The drawing under review shows one solid part. Ordinate dimensions are in mm from its lowest x, y, z. A direction names the side the tool comes from. Round coordinates to 2 decimals unless told otherwise and drop trailing zeros. Order: outer loops, then holes, each group sorted by start corner. A loop starts at its lowest first (then second) coordinate and runs counter-clockwise, first axis right, second up.
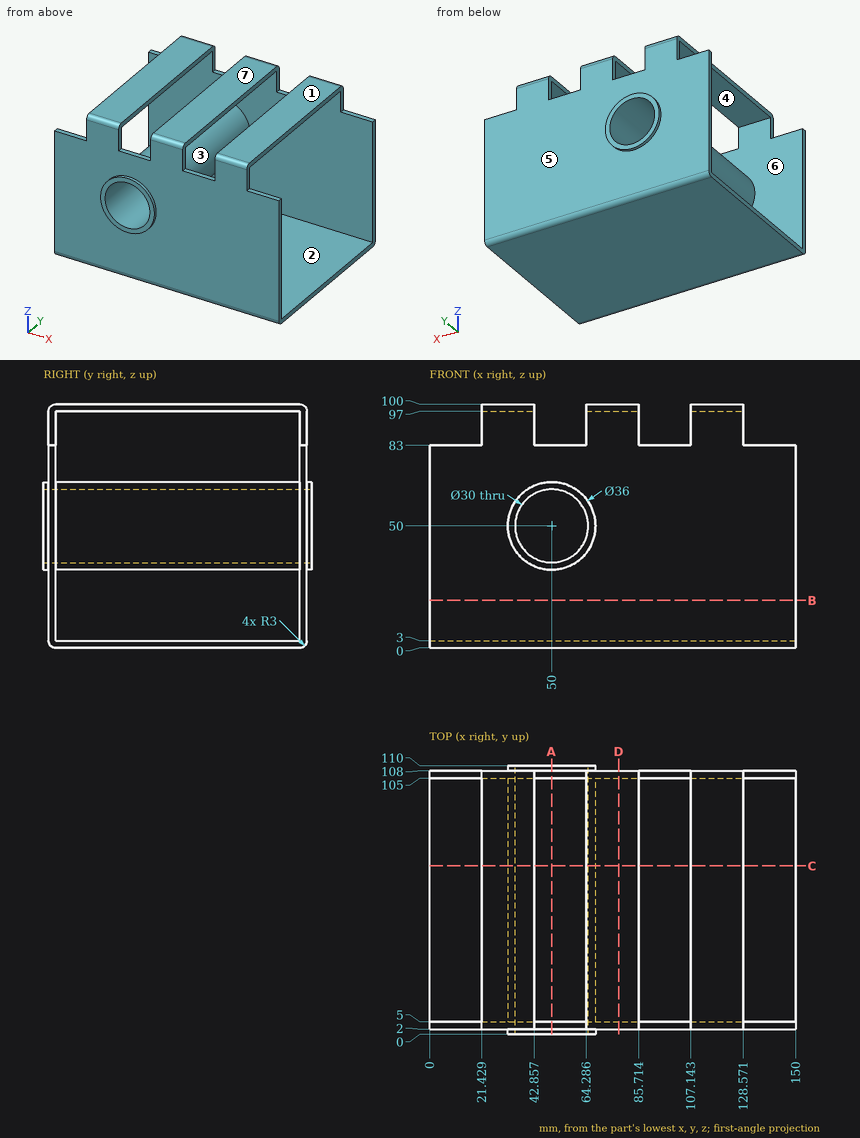
Q1. Clearance check with flat-ended pins moving along their axes: pin 1 (4 mm diameter, centred on x = 40, z = 83, fed in from -Y); pin 2 (1.5 mm diameter, centred on x = 15.5, y = 3.5, fed in from +Z); pin 3 (24 mm diameter, centred on x = 50, z = 50, fed in from -Y); pin 4 (2 mm diameter, centred on y = 56.5, z = 41.5, fed in from -X). State where each tip first meets the part, or that it passes through.
Q2. Wall thickness on line 1 (Z direction, x = 50, y = 41); line 2 (Y direction, x = 89, z = 58); line 3 (Z direction, x = 113.5, y = 45.5): over which ranges is each line inside the solid? List them lowest first.
Q3. Take a section at B-B, the plane z = 19.5. State the section outline as (x, y) points.
Q4. Tool access review of the marked faces 1, 2 and 3: name each direction out of +Z, -Z, +X, -X, +Y, -Y from which nothing blocks a thin tool from reaching the whole face with its end or side.
Q5. Take a section at C-C, the plane y = 69. State the section outline as (x, z) points (1 decimal).
Q6. Mouldability with a two-part tool opening along Y and no side actions: class the marked faces 4, 5, 6 and 7 as +Y half, -Y half, draft (parallel to the pull), parting line (faces both ways), or undercut.
Q7. Take a section at D-D, the plane x = 77.5. State the section outline as (y, z) points, plus the area to 3 significant figures.
Q8. Take a section at A-A, the plane x = 50. State the section outline as (y, z) points, plus the area to 3 significant figures.
Working result:
1. pin 1: stops at y = 2
1. pin 2: stops at z = 83
1. pin 3: passes through
1. pin 4: stops at x = 33.64
2. line 1: z = 0 to 3, 32 to 35, 65 to 68
2. line 2: y = 2 to 5, 105 to 108
2. line 3: z = 0 to 3, 97 to 100
3. outline: (0, 2) - (150, 2) - (150, 5) - (0, 5) - close; (0, 105) - (150, 105) - (150, 108) - (0, 108) - close
4. face 1: +Z, +X, -X, +Y, -Y
4. face 2: +X, -X
4. face 3: none
5. outline: (0, 0) - (150, 0) - (150, 3) - (0, 3) - close; (21.4, 97) - (42.9, 97) - (42.9, 100) - (21.4, 100) - close; circle Ø36 at (50, 50); (64.3, 97) - (85.7, 97) - (85.7, 100) - (64.3, 100) - close; (107.1, 97) - (128.6, 97) - (128.6, 100) - (107.1, 100) - close; hole circle Ø30 at (50, 50)
6. face 4: undercut
6. face 5: +Y half
6. face 6: undercut
6. face 7: draft
7. outline: (2, 3) arc R3 ccw to (5, 0) - (105, 0) arc R3 ccw to (108, 3) - (108, 97) arc R3 ccw to (105, 100) - (5, 100) arc R3 ccw to (2, 97) - close; hole (5, 3) - (105, 3) - (105, 97) - (5, 97) - close
7. area: 1,190 mm2
8. outline: (0, 32) - (2, 32) - (2, 3) arc R3 ccw to (5, 0) - (105, 0) arc R3 ccw to (108, 3) - (108, 32) - (110, 32) - (110, 35) - (0, 35) - close; (0, 65) - (110, 65) - (110, 68) - (108, 68) - (108, 83) - (105, 83) - (105, 68) - (5, 68) - (5, 83) - (2, 83) - (2, 68) - (0, 68) - close; hole (5, 3) - (105, 3) - (105, 32) - (5, 32) - close
8. area: 1,240 mm2
